Can you work these out from the drawing? Everything is in mm from the part's minimum corner. A direction names the side the tool comes from. Give positions to 0.01 mm unless a question says otherwise; leave off trailing zeros. Order: outer loops, then holes, each group sorted by start corner. A loop starts at its lowest first (then second) coordinate and runs counter-clockwise, first axis right, second up. Notation, with made-up numbers: (56.25, -16) - (104.25, -16) arc R14 cw to (104.25, 3) - close; hole circle Ø2 at (25.5, 8). An arc over 180 degrees is marked (long way). Answer as a JSON object with one key per item and string values.
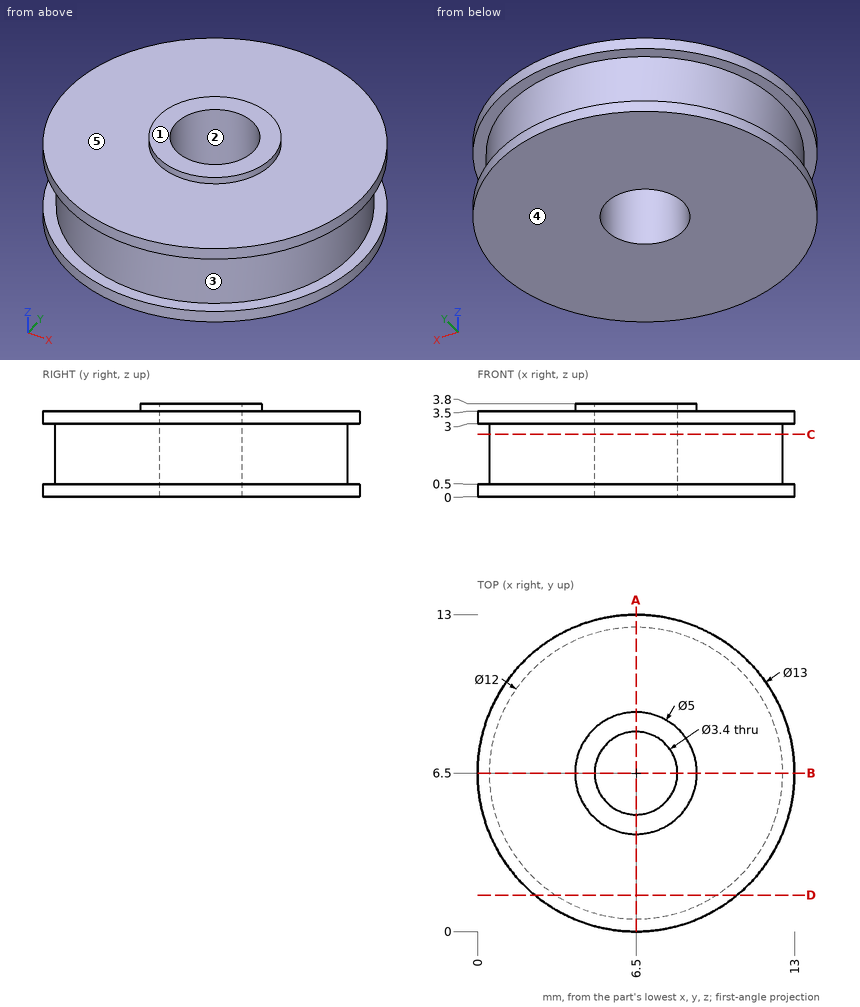
Q1. I need wall thicknesses on L1, parallel to Y at x = 6.5, z = 2.55; L2, parallel to Z at x = 3.25, y = 5.5; L3, parallel to Z at x = 5, y = 0.5. Which ranges of each line are inside material? Lowest first, please.
Recorded:
{"L1": "y = 0.5 to 4.8, 8.2 to 12.5", "L2": "z = 0 to 3.5", "L3": "z = 0 to 0.5, 3 to 3.5"}
Q2. If we section it at A-A, the plane x = 6.5: Please give me the cut outline in (y, z), then the cut area to 3 significant figures.
Recorded:
{"outline": "(0, 0) - (4.8, 0) - (4.8, 3.8) - (4, 3.8) - (4, 3.5) - (0, 3.5) - (0, 3) - (0.5, 3) - (0.5, 0.5) - (0, 0.5) - close; (8.2, 0) - (13, 0) - (13, 0.5) - (12.5, 0.5) - (12.5, 3) - (13, 3) - (13, 3.5) - (9, 3.5) - (9, 3.8) - (8.2, 3.8) - close", "area": "31.6 mm^2"}
Q3. If we section it at C-C, the plane z = 2.55: Please give me the cut outline in (x, y).
Recorded:
{"outline": "circle Ø12 at (6.5, 6.5); hole circle Ø3.4 at (6.5, 6.5)"}
Q4. We'd pull the mould along Y, two halves only. Please class the marked faces 1, 2 and 3: released by +Y, released by -Y, zero draft, split by the parting line, or undercut.
Recorded:
{"face 1": "zero draft", "face 2": "undercut", "face 3": "split by the parting line"}
Q5. Which directions (+Z, -Z, +X, -X, +Y, -Y) give clear straight access to the entire face, cutting with the end or side of a thin tool? Please do the marked faces 4 and 5.
Recorded:
{"face 4": "-Z, +X, -X, +Y, -Y", "face 5": "+Z"}
Q6. If we section it at D-D, the plane y = 1.5: Please give me the cut outline in (x, z).
Recorded:
{"outline": "(2.35, 0) - (10.65, 0) - (10.65, 0.5) - (9.82, 0.5) - (9.82, 3) - (10.65, 3) - (10.65, 3.5) - (2.35, 3.5) - (2.35, 3) - (3.18, 3) - (3.18, 0.5) - (2.35, 0.5) - close"}
